Could you check a few things on this model? Use its own coordinates, in mm. Face numbers are marked on the shaded views. Round coordinates to 2 decimals unless told otherwise and drop trailing zeros. Write each loop counter-clockwise with the first axis right and the second up, starting at its lowest first coordinate (ties: lowest second). Pieces come first, ordered by that corner, then holes. Notation, with made-up numbers: M 34,35 L 73,35 A11 cw 73,45 Z; hole C 44,1 d11. An arc over 180 degrees is marked long. One line per item, written item: value. Start each with the question number.
(1) Thinking about a two-plate mould opening in Z: for the marked faces 1, 2, 3 and 4, which applies, released by +Z, released by -Z, zero draft, split by the parting line, or undercut?
(2) I want a section at C-C on y = 26.5. Please give me the cut outline in (x, z), and give its area (3 significant figures).
(3) I'm going to push flat-ended pins straight in: pin 1 Ø0.5 at (x, z) = (8, 4) entering from +Y; pin 2 Ø0.8 at (x, z) = (-8, 5) entering from +Y; pin 3 Ø1.1 at (x, z) = (0.5, 9) entering from -Y; pin 4 Ø6 at (x, z) = (0, 0) entering from +Y. Where does each tip first touch, or does it pass through?
(4) I want a section at A-A on z = 0. Please give me the cut outline in (x, y).
(5) I want a section at B-B on y = 3.5. Please give me the cut outline in (x, z), and give its area (3 significant figures).
(6) If I drill on L1, parallel to Z at x = 0, y = 28.5; L2, parallel to X at y = 33.5, z = 0.25; L3, parallel to Y at x = -3, z = 4.25, over which ranges is the centre line in solid material (lowest first)?
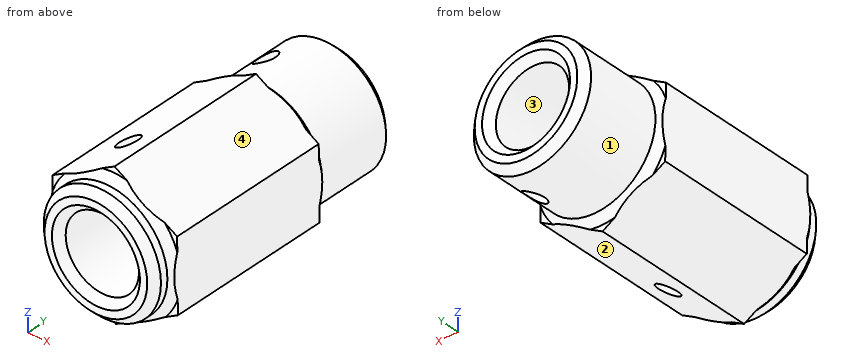
Autodesk Inventor part; units mm, degrees
ref_plane "YZ Plane" through (0, 0, 0) normal (1, 0, 0) x (0, 1, 0)
ref_plane "XZ Plane" through (0, 0, 0) normal (0, 1, 0) x (-1, 0, 0)
ref_plane "XY Plane" through (0, 0, 0) normal (0, 0, 1) x (1, 0, 0)
sketch "Sketch1" plane through (0, 0, 0) normal (0, 1, 0) x (-1, 0, 0)
  line L0 (8.5475, 4.8243) -> (8.4517, -4.9902)
  line L1 (8.4517, -4.9902) -> (-0.0957, -9.8145)
  line L2 (-0.0957, -9.8145) -> (-8.5475, -4.8243)
  line L3 (-8.5475, -4.8243) -> (-8.4517, 4.9902)
  line L4 (-8.4517, 4.9902) -> (0.0957, 9.8145)
  line L5 (0.0957, 9.8145) -> (8.5475, 4.8243)
  circle A0 centre (0, 0) radius 5
  dimension "d0" = 17
  dimension "d1" = 10
extrude "Extrusion1" add sketch "Sketch1" along normal blind 37
sketch "Sketch2" plane through (0, 37, 0) normal (0, 1, 0) x (1, 0, 0)
  circle A0 centre (0, 0) radius 8
  circle A1 centre (0, 0) radius 13
  dimension "d4" = 16
  dimension "d5" = 5
extrude "Extrusion2" cut sketch "Sketch2" against normal blind 12
sketch "Sketch3" plane through (0, 0, 0) normal (0, -1, 0) x (1, 0, 0)
  circle A0 centre (0, 0) radius 8
  circle A1 centre (0, 0) radius 13
  dimension "d9" = 16
  dimension "d10" = 5
extrude "Extrusion3" cut sketch "Sketch3" against normal blind 3
chamfer "Chamfer1" distance 1 angle 45 6 edges at (-8, 3, 0) (-8, 0, 0) (5, 0, 0) (-8, 25, 0) (-8, 37, 0) (5, 37, 0)
ref_plane "Work Plane1" through (0, 31, 0) normal (0, 1, 0) x (1, 0, 0)
sketch "Sketch4" plane through (0, 31, 0) normal (0, 1, 0) x (1, 0, 0)
  line L0 (0, 0) -> (3.9142, 6.6294)
  line L1 (0.0957, 9.8145) -> (0, 0)
  point P0 (8.5475, 4.8243)
  dimension "d20" = 30
ref_plane "Work Plane3" through (4.0674, 31, -6.8889) normal (0.5084234, 0, -0.8611072) x (0, 1, 0)
sketch "Sketch6" plane through (4.0674, 31, -6.8889) normal (0.5084234, 0, -0.8611072) x (0, 1, 0)
  circle A0 centre (0, 0) radius 1.5
  point P0 (-31, 0)
  dimension "d16" = 3
extrude "Extrusion4" cut sketch "Sketch6" against normal through all
sketch "Sketch9" plane through (0.0957, 3, -9.8145) normal (0.5084234, 0, -0.8611072) x (-0.8611072, 0, -0.5084234)
  circle A0 centre (-4.9075, 7) radius 1.5
  line L0 (-9.815, 0) -> (-9.815, 22)
  line L1 (0, 0) -> (0, 22)
  point P0 (-4.9075, -3)
  dimension "d31" = 3
  dimension "d32" = 9.8149
  dimension "d33" = 4.9075
  dimension "d34" = 10
extrude "Extrusion5" cut sketch "Sketch9" against normal through all
thread "Thread2"
equation "\"d33\" = 0.5 * d32"
properties part number "AnyaKicsi"
Found:
1. face 1: split by the parting line
1. face 2: released by -Z
1. face 3: undercut
1. face 4: released by +Z
2. outline: C 0,0 d16; hole C 0,0 d10
2. area: 123 mm²
3. pin 1: stops at y = 25.31
3. pin 2: stops at y = 25
3. pin 3: stops at y = 2.46
3. pin 4: passes through
4. outline: M -8.5,2.5 L -8,2 L -8,1 L -7,0 L -6,0 L -5,1 L -5,36 L -6,37 L -7,37 L -8,36 L -8,26 L -8.5,25.5 Z; M 5,1 L 6,0 L 7,0 L 8,1 L 8,2 L 8.5,2.5 L 8.5,25.5 L 8,26 L 8,36 L 7,37 L 6,37 L 5,36 Z
5. outline: M -8.55,4.82 L -8.45,-4.99 L 0.1,-9.81 L 8.55,-4.82 L 8.45,4.99 L -0.1,9.81 Z; hole C 0,0 d10
5. area: 172 mm²
6. L1: z = -8 to -5, 5 to 8
6. L2: x = -8 to -4.99, 4.99 to 8
6. L3: y = 0.8 to 8.56, 11.44 to 29.56, 32.44 to 36.2
